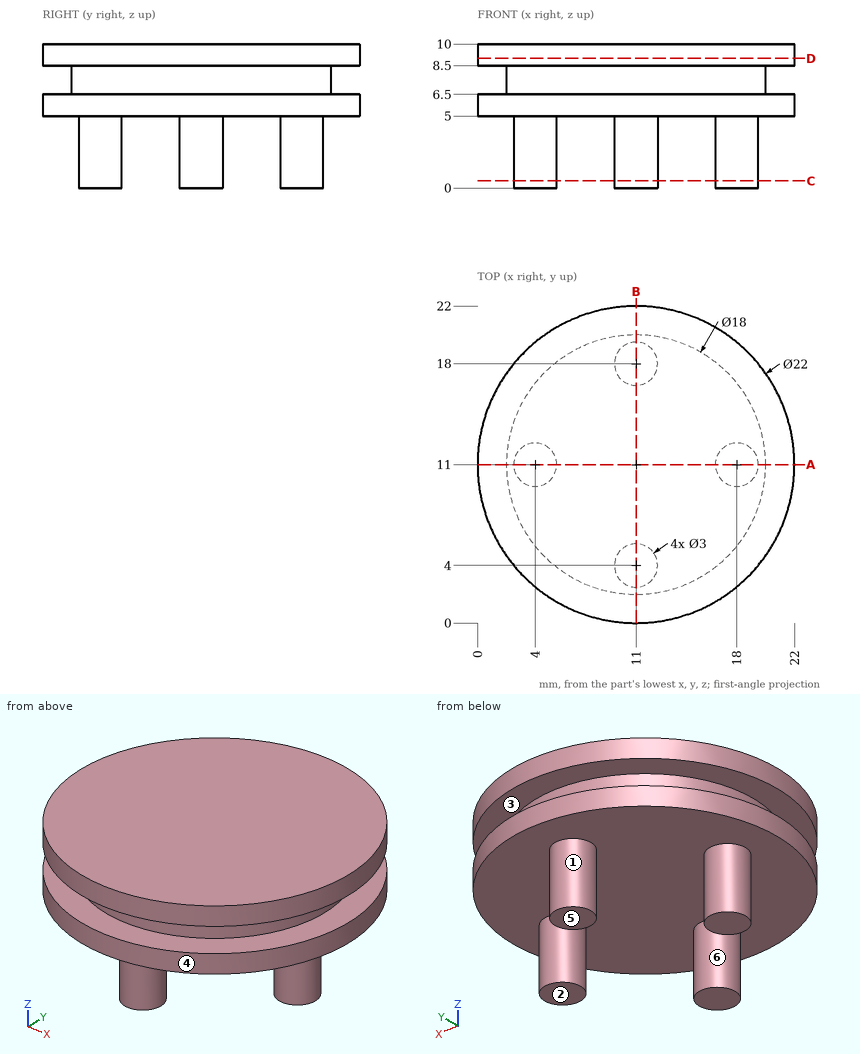
Part print with two shaded views. Sizes in mm from the minimum x, y, z corner. A direction names the side the tool comes from. Round coordinates to 2 decimals unless told otherwise and drop trailing zeros. Order: outer loops, then holes, each group sorted by start corner. A loop starts at its lowest first (then second) coordinate and runs counter-clockwise, first axis right, second up. Notation, with made-up numbers: M 25.5,-8.75 L 65.5,-8.75 A15 cw 65.5,15.25 Z; hole C 59.25,60 d8. An arc over 180 degrees is marked long. Answer in a Markdown table with one row per item. Add a question column.
Q1. Cut at C-C on z = 0.5. Give the cut face in (x, y).
Q2. Cut at A-A on y = 11. Give the cut face in (x, z), and give its area (3 significant figures).
Q3. Pin check, flat tips, straight feed: pin 1 (4 mm diameter, centred on y = 3, z = 5.5, fed in from -X); pin 2 (5 mm diameter, centred on y = 16.5, z = 7.5, fed in from +X); pin 3 (2 mm diameter, centred on x = 4.5, z = 7, fed in from +Y). Stop position of each tip, or through.
Q4. Cut at D-D on z = 9. Give the cut face in (x, y).
Q5. 3-axis set-ups, long thin cutter, end or side, ignore diameter. For the marked faces 1, 2 and 3: which of +Z, -Z, +X, -X, +Y, -Y reach the whole face in a straight line?
Q6. Mould opens along Y. For the marked faces 4, 5 and 6 say: +Y half, -Y half, draft (parallel to the pull), parting line (faces both ways), or undercut.
Q7. Wall check: L1, parallel to Z at x = 2, y = 14.5; L2, parallel to Z at x = 5, y = 16.75; L3, parallel to Y at x = 11.75, z = 2. Give the ranges that are in metal, low to high. Write a range as from..to.
Established:
| question | item | result |
|---|---|---|
| 1 | outline | C 4,11 d3; C 11,4 d3; C 11,18 d3; C 18,11 d3 |
| 2 | outline | M 0,5 L 2.5,5 L 2.5,0 L 5.5,0 L 5.5,5 L 16.5,5 L 16.5,0 L 19.5,0 L 19.5,5 L 22,5 L 22,6.5 L 20,6.5 L 20,8.5 L 22,8.5 L 22,10 L 0,10 L 0,8.5 L 2,8.5 L 2,6.5 L 0,6.5 Z |
| 2 | area | 132 mm2 |
| 3 | pin 1 | stops at x = 1.78 |
| 3 | pin 2 | stops at x = 21.52 |
| 3 | pin 3 | stops at y = 20.45 |
| 4 | outline | C 11,11 d22 |
| 5 | face 1 | -Z |
| 5 | face 2 | -Z, +X, -X, +Y, -Y |
| 5 | face 3 | none |
| 6 | face 4 | parting line |
| 6 | face 5 | draft |
| 6 | face 6 | undercut |
| 7 | L1 | z = 5..6.5, 8.5..10 |
| 7 | L2 | z = 5..10 |
| 7 | L3 | y = 2.7..5.3, 16.7..19.3 |
